The model under review builds one solid part; all positions refer to its coordinate system, in mm. A direction names the side the tool comes from. Round coordinates to 2 decimals unless told otherwise and drop trailing zeros. Loops run counter-clockwise (first coordinate to the right, second up) from the corner with the lowest first, then second, coordinate; pieces in that order, holes last. Notation, with made-up numbers: (3, -31) -> (55, -31) arc R10 cw to (55, -17) -> close; hole circle Ø4 at (43, 50). An arc over 180 degrees is marked (long way). Use a Markdown table: item, result. Add a question column.
1) Mouldability with a two-part tool opening along Y and no side actions: class faces 1 (the flat face through (142.5, -1, 12)), 2 (the flat face through (2, -1, 4)), 3 (the flat face through (147.5, 1, 10)), 4 (the flat face through (-2, 52.3, 10)) as released by +Y, released by -Y, zero draft, split by the parting line, or undercut.
2) Insertion check: pin 1 (1.6 mm diameter, centred on x = 48, y = -37.9, fed in from +Z); pin 2 (1.1 mm diameter, centred on x = 117.55, y = 19.4, fed in from +Z). Each pin has a flat end and moves straight along its axis. Give the tip position at first contact, or say it passes through.
3) Consider section A-A on x = 18. Give the boundary of the cut face in (y, z), plus the area to 3 significant figures.
4) Wall thickness on probe 1 along Y at (x, z) = (-14.5, 6.65) (3 decimals); probe 2 along X at (y, z) = (-9.2, 5.4) (3 decimals); probe 3 along X at (y, z) = (0.3, 5) (3 decimals): over which ranges is each line inside the solid? List them lowest first.
5) For faces 5 (the flat face through (-142.5, 1, 12)), 6 (the flat face through (-44, 51, 20)), 7 (the flat face through (-124, 50, 5.69)), list the 3-axis set-ups (+Z, -Z, +X, -X, +Y, -Y) from which the entire face can be reached by the end or side of a thin tool; tool diameter is ignored.
6) Consider section B-B on y = 40. Give the boundary of the cut face in (x, z), plus the area to 3 significant figures.
Autodesk Fusion 360 part; units mm, degrees
sketch "Body" plane through (0, 0, 0) normal (0, 0, 1) x (1, 0, 0)
  line L0 (147.5, -52.3) -> (-147.5, -52.3)
  line L1 (-147.5, -52.3) -> (-147.5, 52.3)
  line L2 (-147.5, 52.3) -> (147.5, 52.3)
  line L3 (147.5, 52.3) -> (147.5, -52.3)
  line L4 (147.5, -52.3) -> (-147.5, 52.3) construction
  line L5 (-147.5, -52.3) -> (147.5, 52.3) construction
  dimension "d15" = 295
  dimension "d16" = 104.6
extrude "Extrude3" add sketch "Body" along normal blind 20
sketch "Walls" plane through (0, 0, 20) normal (0, 0, 1) x (-1, 0, 0)
  line L0 (-147.5, -52.3) -> (147.5, -52.3)
  line L1 (147.5, -52.3) -> (147.5, 52.3)
  line L2 (147.5, 52.3) -> (-147.5, 52.3)
  line L3 (-147.5, 52.3) -> (-147.5, -52.3)
  line L4 (142.5, 47.3) -> (-142.5, 47.3)
  line L5 (-142.5, 47.3) -> (-142.5, -47.3)
  line L6 (-142.5, -47.3) -> (142.5, -47.3)
  line L7 (142.5, -47.3) -> (142.5, 47.3)
  dimension "d19" = -5
extrude "Extrude4" cut sketch "Walls" against normal up to surface (16 mm away) contours L4 L5 L6 L7
sketch "Screws" plane through (0, 0, 4) normal (0, 0, 1) x (-1, 0, 0)
  line L0 (142.5, 47.3) -> (-142.5, 47.3)
  line L1 (-142.5, 47.3) -> (-142.5, -47.3)
  line L2 (-142.5, -47.3) -> (142.5, -47.3)
  line L3 (142.5, -47.3) -> (142.5, 47.3)
  circle A0 centre (117.3, -19.4) radius 1.625
  circle A1 centre (140.5, 9.2) radius 1.625
  circle A2 centre (14.5, -0.3) radius 1.625
  circle A3 centre (-48, 37.9) radius 1.625
  circle A4 centre (-117.55, -19.4) radius 1.625
  circle A5 centre (-140.5, 9.2) radius 1.625
  circle A6 centre (140.5, 9.2) radius 0.625
  circle A7 centre (117.3, -19.4) radius 0.625
  circle A8 centre (14.5, -0.3) radius 0.625
  circle A9 centre (-48, 37.9) radius 0.625
  circle A10 centre (-117.55, -19.4) radius 0.625
  circle A11 centre (-140.5, 9.2) radius 0.625
  point P0 (117.3, -19.4)
  dimension "d32" = 3.25
  dimension "d33" = 27.9
  dimension "d34" = 25.2
  dimension "d35" = 3.25
  dimension "d36" = 2
  dimension "d37" = 56.5
  dimension "d38" = 3.25
  dimension "d39" = 128
  dimension "d40" = 47
  dimension "d41" = 3.25
  dimension "d42" = 85.2
  dimension "d43" = 190.5
  dimension "d44" = 3.25
  dimension "d45" = 27.9
  dimension "d46" = 24.95
  dimension "d47" = 3.25
  dimension "d48" = 56.5
  dimension "d49" = 2
  dimension "d57" = -1
  dimension "d58" = -1
  dimension "d59" = -1
  dimension "d60" = -1
  dimension "d61" = -1
  dimension "d62" = -1
extrude "Extrude9" add sketch "Screws" along normal blind 5 contours A0 | A1 | A2 | A3 | A4 | A5
fillet "Fillet1" [suppressed]
thread "Thread2" [suppressed]
sketch "Sketch13" plane through (0, 47.3, 0) normal (0, -1, 0) x (1, 0, 0)
  line L0 (-142.5, 4) -> (142.5, 4)
  line L1 (142.5, 4) -> (142.5, 20)
  line L2 (142.5, 20) -> (-142.5, 20)
  line L3 (-142.5, 20) -> (-142.5, 4)
  line L4 (-119.83, 9) -> (-128.77, 9)
  line L5 (-128.77, 9) -> (-128.77, 5.69)
  line L6 (-128.77, 5.69) -> (-119.83, 5.69)
  line L7 (-119.83, 5.69) -> (-119.83, 9)
  line L8 (-119.83, 9) -> (-128.77, 5.69) construction
  line L9 (-128.77, 9) -> (-119.83, 5.69) construction
  line L10 (142.5, 4) -> (-142.5, 4)
  point P0 (-124.3, 7.345)
  dimension "d65" = 8.94
  dimension "d66" = 3.31
  dimension "d67" = 18.2
  dimension "d71" = 5
extrude "Extrude10" cut sketch "Sketch13" against normal up to surface (5 mm away) contours L4 L5 L6 L7
fillet "Fillet3" [suppressed]
equation "d15 = 285 mm + 10 mm"
equation "d16 = 94.6 mm + 10 mm"
equation "d32 = 2 mm + 1.25 mm"
equation "d67 = 25.2 mm - 7 mm"
equation "d73 = ( 3.31 / 2 ) * 1 mm"
Result set:
| question | item | result |
|---|---|---|
| 1 | face 1 | undercut |
| 1 | face 2 | undercut |
| 1 | face 3 | zero draft |
| 1 | face 4 | released by +Y |
| 2 | pin 1 | z = 9 |
| 2 | pin 2 | z = 4 |
| 3 | outline | (-52.3, 0) -> (52.3, 0) -> (52.3, 20) -> (47.3, 20) -> (47.3, 4) -> (-47.3, 4) -> (-47.3, 20) -> (-52.3, 20) -> close |
| 3 | area | 578 mm2 |
| 4 | probe 1 | -52.3 to -47.3, -1.325 to -0.325, 0.925 to 1.925, 47.3 to 52.3 |
| 4 | probe 2 | -147.5 to -142.5, -142.125 to -141.125, -139.875 to -138.875, 138.875 to 139.875, 141.125 to 142.125, 142.5 to 147.5 |
| 4 | probe 3 | -147.5 to -142.5, -16.125 to -15.125, -13.875 to -12.875, 142.5 to 147.5 |
| 5 | face 5 | +Z |
| 5 | face 6 | +Z, +X, -X, +Y, -Y |
| 5 | face 7 | +Y |
| 6 | outline | (-147.5, 0) -> (147.5, 0) -> (147.5, 20) -> (142.5, 20) -> (142.5, 4) -> (-142.5, 4) -> (-142.5, 20) -> (-147.5, 20) -> close |
| 6 | area | 1,340 mm2 |
